from build123d import *

# Parameters (mm, degrees)
F1_DEPTH    = 60
F2_T1_DEPTH = 130.2639714598
F2_T4_ANGLE = 327.2570469478
F3_R        = 7.5
F4_DEPTH    = 25


# Not quite as in the source:
# - a fillet or chamfer that OpenCascade refuses, or shapes differently, is made with other operations: its cross-section is extruded or revolved along the edge and cut away or added


with BuildPart() as f1:
    # F0 (on Front) → F1 (new body)
    with BuildSketch(Plane.XZ):
        with BuildLine():
            Line((15.8661792875, 46.7765345339), (7.8661792875, 46.7765345339))
            Line((7.8661792875, 46.7765345339), (7.8661792875, -40.0019907292))
            ThreePointArc((7.8661792875, -40.0019907292), (3.8517652045, -52.021185498), (-6.5799250014, -59.2153777921))
            Line((-6.5799250014, -59.2153777921), (-46.7759604719, -70.834598717))
            Line((-46.7759604719, -70.834598717), (-55.08180854, -79.3164507385))
            Line((-55.08180854, -79.3164507385), (0, -64.9890005589))
            ThreePointArc((0, -64.9890005589), (9.4773105279, -59.0361843334), (15.8661792875, -49.8471804794))
            Line((15.8661792875, -49.8471804794), (15.8661792875, -40.0019907292))
            Line((15.8661792875, -40.0019907292), (15.8661792875, 46.7765345339))
        make_face()
    extrude(amount=F1_DEPTH)

    # F2: chamfer of 6 x 34.0276909177 on 2 edges, made by hand

    # F2_s2 → F2_t1 (cut)
    with BuildSketch(Plane(origin=(-21.8695743552, 0, -6.3217034464), x_dir=(0, 1, 0), z_dir=(-0.9606693531, 0, -0.2776947856))):
        Polygon((-60, 61.0591878178), (-25.9723090823, 55.0591878178), (-60, 55.0591878178), align=None)
    extrude(amount=F2_T1_DEPTH, mode=Mode.SUBTRACT)

    # F2_s3 → F2_t4 (revolve, cut)
    with BuildSketch(Plane(origin=(-0.1774752696, 0, 0.0529760926), x_dir=(0, 1, 0), z_dir=(0.9582213809, 0, -0.2860275953))):
        Polygon((-60, -67.8013703537), (-25.9723090823, -61.8013703537), (-60, -61.8013703537), align=None)
    revolve(axis=Axis((-12.1338207125, -60, -40.0019907292), (0, 1, 0)), revolution_arc=F2_T4_ANGLE, mode=Mode.SUBTRACT)

    # F3 (on face) → F4 (cut)
    with BuildSketch(Plane(origin=(7.8661792875, 0, 0), x_dir=(0, -1, 0), z_dir=(-1, 0, 0))):
        with Locations((30, 28.4848585725)):
            Circle(F3_R)
    extrude(amount=-F4_DEPTH, mode=Mode.SUBTRACT)


solid = f1.part
The listing builds one solid part. Answer for the finished solid, in the listing's coordinates (mm). A direction names the side the tool comes from. Give positions to 0.01 mm unless a question says otherwise; leave off trailing zeros. Loops run counter-clockwise (first coordinate to the right, second up) from the corner with the lowest first, then second, coordinate; pieces in that order, holes last.
Item 1: A cutting plane is placed at A-A (z = 31.5). Give the vertices of the cut face in (x, y).
Derived:
outline: (7.87, -60) - (15.87, -60) - (15.87, -36.87) - (7.87, -36.87) - close; (7.87, -23.13) - (15.87, -23.13) - (15.87, 0) - (7.87, 0) - close
Item 2: Find the intervals of material crossed by line 1 along Z through (x, y) = (13.75, -30); line 2 along Z through (x, y) = (10.75, -30); line 3 along X through (y, z) = (-56.5, 32), in increasing order.
Derived:
line 1: z = -53.84 to 20.98, 35.98 to 46.78
line 2: z = -57.74 to 20.98, 35.98 to 46.78
line 3: x = 7.87 to 15.87
Item 3: Each of these flat-tipped pins is pushed along its axis until it touches: pin 1 Ø4 at (x, y) = (-9, -45.5) entering from -Z; pin 2 Ø1.5 at (y, z) = (-46.5, -53) entering from -X; pin 3 Ø2 at (x, y) = (-14.5, -15) entering from +Z. Where does it stop, or does it pass through?
Derived:
pin 1: stops at z = -67.85
pin 2: stops at x = 7.05
pin 3: stops at z = -61.22
Item 4: A cutting plane is placed at D-D (x = -23.5). Give the vertices of the cut face in (y, z).
Derived:
outline: (-60, -71.1) - (0, -71.1) - (0, -64.11) - (-25.97, -64.11) - (-60, -70.35) - close
Item 5: Determine the mould class of faces 3 (the flat face through (-51.794, -22.571, -75.959)), 4 (the flat face through (9, 0, -25)), 5 (the conical face through (9.903, -42.748, -46.44)) for opening direction Z: +Z half, -Z half, draft (parallel to the pull), parting line (faces both ways), or undercut.
Derived:
face 3: +Z half
face 4: draft
face 5: undercut
Item 6: A cutting plane is placed at B-B (y = -30). Give the vertices of the cut face in (x, z) (3 decimals), then the cut area to 3 significant figures.
Derived:
outline: (-55.082, -79.316) - (0, -64.989) arc R28 ccw to (15.866, -49.847) - (15.866, 20.985) - (7.866, 20.985) - (7.866, -34.625) arc R20.71 cw to (-6.383, -59.898) - (-47.786, -71.866) - close; (7.866, 35.985) - (15.866, 35.985) - (15.866, 46.777) - (7.866, 46.777) - close
area: 1,100 mm2
Item 7: A tool of negligible diameter and unlimited length cuts with its end or side. For faces 1 (the cylindrical face through (9.363, -29.58, -59.145)), 2 (the flat face through (7.866, -30, 4)), from which of +Z, -Z, +X, -X, +Y, -Y can it reach the whole face along a straight path? Write none if from no direction.
Derived:
face 1: -Z, +X, +Y, -Y
face 2: +Z, -X, +Y, -Y
Item 8: A cutting plane is placed at C-C (y = -12). Give the vertices of the cut face in (x, z).
Derived:
outline: (-55.08, -79.32) - (0, -64.99) arc R28 ccw to (15.87, -49.85) - (15.87, 46.78) - (7.87, 46.78) - (7.87, -40) arc R20 cw to (-6.58, -59.22) - (-46.78, -70.83) - close
